```python
from build123d import *

# Parameters (mm, degrees)
EXTRUSION_DEPTH = 4.7625
CHAMFER1_SIZE   = 0.635


with BuildPart() as part:
    # profile → extrusion (new body, symmetric)
    with BuildSketch(Plane.XY):
        with BuildLine():
            Line((-0.396875, 4.745934732), (-0.396875, 11.105410685))
            ThreePointArc((-0.396875, 11.105410685), (0, -11.1125), (0.396875, 11.105410685))
            Line((0.396875, 11.105410685), (0.396875, 4.745934732))
            ThreePointArc((0.396875, 4.745934732), (0, -4.7625), (-0.396875, 4.745934732))
        make_face()
    extrude(amount=EXTRUSION_DEPTH, both=True)

    # Chamfer1
    chamfer1_edges = [part.edges().sort_by_distance(p)[0] for p in [
        (0, -11.1125, 4.7625),
        (0, -11.1125, -4.7625),
    ]]
    chamfer(chamfer1_edges, length=CHAMFER1_SIZE)


solid = part.part
```
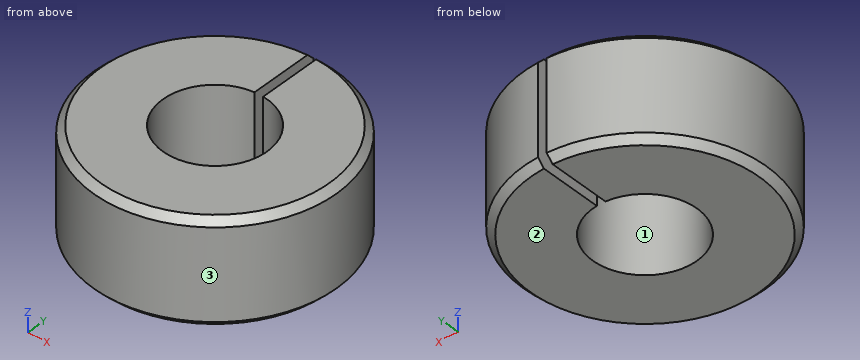
The listing builds one solid part. Answer for the finished solid, in the listing's coordinates (mm). Face numbers are marked on the shaded views. Round coordinates to 2 decimals unless told otherwise and drop trailing zeros. Write each loop counter-clockwise with the first axis right and the second up, starting at its lowest first coordinate (ties: lowest second). Pieces come first, ordered by that corner, then holes. Notation, with made-up numbers: (-15, -15.75) -> (-7, -15.75) arc R20 ccw to (-7, -0.75) -> close; hole circle Ø4 at (40, 14.5). An arc over 180 degrees is marked (long way). Use CSV: the item, a comma, the result in double quotes. Start each with the question number.
(1) Section B-B on x = 0 is taken. Give the vertices of the cut face in (y, z).
(2) Section C-C on z = 3.5 is taken. Give the vertices of the cut face in (x, y) (1 decimal).
(3) The mould has two halves that part along Y. Classify the marked faces 1, 2 and 3: released by +Y, released by -Y, zero draft, split by the parting line, or undercut.
(4) Each of these flat-tipped pins is pushed along its axis until it touches: pin 1 (5 mm diameter, centred on y = 6.5, z = 1.5, fed in from -X); pin 2 (3 mm diameter, centred on y = 4, z = 3, fed in from +X); pin 3 (8.5 mm diameter, centred on x = 0, y = 0, fed in from +Z); pin 4 (1 mm diameter, centred on x = -1.5, z = -3, fed in from -Y). Where does it stop, or does it pass through?
(5) Consider L1, parallel to X at y = 0, z = 2.25; L2, parallel to Y at x = 2.25, z = 3.5; L3, parallel to X at y = 1.5, z = 1.75. Determine where each line is inside the solid, lowest interval first. Write a range as from..to.
(6) Section A-A on y = 0 is taken. Give the vertices of the cut face in (x, z), then the cut area to 3 significant figures.
A:
1,outline,"(-11.11, -4.13) -> (-10.48, -4.76) -> (-4.76, -4.76) -> (-4.76, 4.76) -> (-10.48, 4.76) -> (-11.11, 4.13) -> close"
2,outline,"(-0.4, 4.7) -> (-0.4, 11.1) arc R11.1 ccw (long way) to (0.4, 11.1) -> (0.4, 4.7) arc R4.8 cw (long way) to start"
3,face 1,"undercut"
3,face 2,"zero draft"
3,face 3,"split by the parting line"
4,pin 1,"stops at x = -10.37"
4,pin 2,"stops at x = 10.83"
4,pin 3,"passes through"
4,pin 4,"stops at y = -11.07"
5,L1,"x = -11.11..-4.76, 4.76..11.11"
5,L2,"y = -10.88..-4.2, 4.2..10.88"
5,L3,"x = -11.01..-4.52, 4.52..11.01"
6,outline,"(-11.11, -4.13) -> (-10.48, -4.76) -> (-4.76, -4.76) -> (-4.76, 4.76) -> (-10.48, 4.76) -> (-11.11, 4.13) -> close; (4.76, -4.76) -> (10.48, -4.76) -> (11.11, -4.13) -> (11.11, 4.13) -> (10.48, 4.76) -> (4.76, 4.76) -> close"
6,area,"120 mm²"
